```python
from build123d import *

# Parameters (mm, degrees)
SKETCH1_R           = 60
BOSS_EXTRUDE1_DEPTH = 9.652
SKETCH2_R           = 4
BOSS_EXTRUDE2_DEPTH = 25.4
SKETCH3_R           = 60
BOSS_EXTRUDE3_DEPTH = 20
SKETCH5_R           = 36
CUT_EXTRUDE1_DEPTH  = 92.807639682
SKETCH6_R           = 47.5
CUT_EXTRUDE2_DEPTH  = 10
FILLET1_R           = 2.54


with BuildPart() as part:
    # Sketch1 → Boss-Extrude1 (new body)
    with BuildSketch(Plane(origin=(0, 0, 0), x_dir=(1, 0, 0), z_dir=(0, 1, 0))):
        with Locations(Location((0, 0, 0), (0, 0, 270))):
            Circle(SKETCH1_R)
        with BuildLine():
            ThreePointArc((-10.16, 30.080506977), (0, 22.86), (10.16, 30.080506977))
            ThreePointArc((10.16, 30.080506977), (15.875, 27.49630657), (20.970483201, 23.839071591))
            ThreePointArc((20.970483201, 23.839071591), (19.797340731, 11.43), (31.130483201, 6.241435386))
            ThreePointArc((31.130483201, 6.241435386), (31.75, 0), (31.130483201, -6.241435386))
            ThreePointArc((31.130483201, -6.241435386), (19.797340731, -11.43), (20.970483201, -23.839071591))
            ThreePointArc((20.970483201, -23.839071591), (15.875, -27.49630657), (10.16, -30.080506977))
            ThreePointArc((10.16, -30.080506977), (0, -22.86), (-10.16, -30.080506977))
            ThreePointArc((-10.16, -30.080506977), (-15.875, -27.49630657), (-20.970483201, -23.839071591))
            ThreePointArc((-20.970483201, -23.839071591), (-19.797340731, -11.43), (-31.130483201, -6.241435386))
            ThreePointArc((-31.130483201, -6.241435386), (-31.75, 0), (-31.130483201, 6.241435386))
            ThreePointArc((-31.130483201, 6.241435386), (-19.797340731, 11.43), (-20.970483201, 23.839071591))
            ThreePointArc((-20.970483201, 23.839071591), (-15.875, 27.49630657), (-10.16, 30.080506977))
        make_face(mode=Mode.SUBTRACT)
    extrude(amount=BOSS_EXTRUDE1_DEPTH)

    # Sketch2 → Boss-Extrude2 (add)
    with BuildSketch(Plane(origin=(0, 9.652, 0), x_dir=(1, 0, 0), z_dir=(0, 1, 0))):
        with Locations(Location((0, 45, 0), (0, 0, 270))):
            Circle(SKETCH2_R)
        with Locations(Location((38.97114317, -22.5, 0), (0, 0, 270))):
            Circle(SKETCH2_R)
        with Locations(Location((-38.97114317, -22.5, 0), (0, 0, 270))):
            Circle(SKETCH2_R)
    extrude(amount=BOSS_EXTRUDE2_DEPTH)

    # Sketch3 → Boss-Extrude3 (add)
    with BuildSketch(Plane(origin=(0, 35.052, 0), x_dir=(1, 0, 0), z_dir=(0, 1, 0))):
        with Locations(Location((0, 0, 0), (0, 0, 270))):
            Circle(SKETCH3_R)
    extrude(amount=BOSS_EXTRUDE3_DEPTH)

    # Sketch5 → Cut-Extrude1 (cut, through all)
    with BuildSketch(Plane.XZ.offset(-35.052)):
        with Locations(Location((0, 0, 0), (0, 0, 270))):
            Circle(SKETCH5_R)
    extrude(amount=-CUT_EXTRUDE1_DEPTH, mode=Mode.SUBTRACT)

    # Sketch6 → Cut-Extrude2 (cut)
    with BuildSketch(Plane(origin=(0, 55.052, 0), x_dir=(1, 0, 0), z_dir=(0, 1, 0))):
        with Locations(Location((0, 0, 0), (0, 0, 270))):
            Circle(SKETCH6_R)
    extrude(amount=-CUT_EXTRUDE2_DEPTH, mode=Mode.SUBTRACT)

    # Fillet1
    fillet1_edges = [part.edges().sort_by_distance(p)[0] for p in [
        (-10.16, 4.826, 30.080506977),
        (10.16, 4.826, 30.080506977),
        (20.970483201, 4.826, 23.839071591),
        (31.130483201, 4.826, 6.241435386),
        (31.130483201, 4.826, -6.241435386),
        (20.970483201, 4.826, -23.839071591),
        (10.16, 4.826, -30.080506977),
        (-10.16, 4.826, -30.080506977),
        (-20.970483201, 4.826, -23.839071591),
        (-31.130483201, 4.826, -6.241435386),
        (-31.130483201, 4.826, 6.241435386),
        (-20.970483201, 4.826, 23.839071591),
    ]]
    fillet(fillet1_edges, radius=FILLET1_R)


solid = part.part
```
For this review, take the finished solid that the model builds, in its own axes (mm). A direction names the side the tool comes from. Coordinates: 2 decimals unless noted, no trailing zeros. Order: outer loops, then holes, each group sorted by start corner. A loop starts at its lowest first (then second) coordinate and runs counter-clockwise, first axis right, second up. Notation, with made-up numbers: (75.25, 24) -> (89.25, 24) arc R9 cw to (89.25, 28) -> close; hole circle Ø11 at (-1.5, -26.75). An arc over 180 degrees is marked (long way). Answer as CSV lines item,"result".
Q1. We need section D-D (x = -26.5). State the section outline as (y, z) points, plus the area to 3 significant figures.
Model answer:
outline,"(0, -53.83) -> (9.65, -53.83) -> (9.65, -6.37) -> (0, -6.37) -> close; (0, 6.37) -> (9.65, 6.37) -> (9.65, 53.83) -> (0, 53.83) -> close; (35.05, -53.83) -> (55.05, -53.83) -> (55.05, -39.42) -> (45.05, -39.42) -> (45.05, -24.37) -> (35.05, -24.37) -> close; (35.05, 24.37) -> (45.05, 24.37) -> (45.05, 39.42) -> (55.05, 39.42) -> (55.05, 53.83) -> (35.05, 53.83) -> close"
area,"1,790 mm2"
Q2. For faces 1 (the face through (-2.4, 22.2, -48.2)), 2 (the face through (-0.16, 4.76, -22.86)), 3 (the face through (10.81, 39.98, -34.34)), list the 3-axis set-ups (+Z, -Z, +X, -X, +Y, -Y) from which the entire face can be reached by the end or side of a thin tool; tool diameter is ignored.
Model answer:
face 1,"none"
face 2,"+Y, -Y"
face 3,"+Y"
Q3. Clearance check with flat-ended pins moving along their axes: pin 1 Ø1.5 at (y, z) = (49.5, 45.5) entering from +X; pin 2 Ø10 at (y, z) = (24, 14.5) entering from -X; pin 3 Ø4 at (x, y) = (-20.5, 45) entering from +Z. State where each tip first meets the part, or that it passes through.
Model answer:
pin 1,"stops at x = 39.97"
pin 2,"stops at x = -41.62"
pin 3,"stops at z = 57.08"
Q4. We need section C-C (z = 0). State the section outline as (x, y) points.
Model answer:
outline,"(-60, 0) -> (-31.75, 0) -> (-31.75, 9.65) -> (-60, 9.65) -> close; (-60, 35.05) -> (-36, 35.05) -> (-36, 45.05) -> (-47.5, 45.05) -> (-47.5, 55.05) -> (-60, 55.05) -> close; (31.75, 0) -> (60, 0) -> (60, 9.65) -> (31.75, 9.65) -> close; (36, 35.05) -> (60, 35.05) -> (60, 55.05) -> (47.5, 55.05) -> (47.5, 45.05) -> (36, 45.05) -> close"
Q5. Draft analysis for pull direction X (two halves, no side actions). For faces 4 (the face through (18.1, 55.052, 44.2)), 5 (the face through (-38.795, 22.174, 18.504)), 6 (the face through (2.64, 4.76, -59.94)), state which applies: released by +X, released by -X, zero draft, split by the parting line, or undercut.
Model answer:
face 4,"zero draft"
face 5,"undercut"
face 6,"split by the parting line"
Q6. Wall thickness on line 1 along X through (y, z) = (5, 0); line 2 along Y through (x, z) = (-25.5, -53.5); line 3 along X through (y, z) = (38, 0): over which ranges is each line inside the solid? List them lowest first. Write a range as [from, to].
Model answer:
line 1,"x = [-60, -31.75], [31.75, 60]"
line 2,"y = [0, 9.65], [35.05, 55.05]"
line 3,"x = [-60, -36], [36, 60]"
Q7. We need section A-A (x = 0). State the section outline as (y, z) points.
Model answer:
outline,"(0, -60) -> (9.65, -60) -> (9.65, -49) -> (35.05, -49) -> (35.05, -60) -> (55.05, -60) -> (55.05, -47.5) -> (45.05, -47.5) -> (45.05, -36) -> (35.05, -36) -> (35.05, -41) -> (9.65, -41) -> (9.65, -22.86) -> (0, -22.86) -> close; (0, 22.86) -> (9.65, 22.86) -> (9.65, 60) -> (0, 60) -> close; (35.05, 36) -> (45.05, 36) -> (45.05, 47.5) -> (55.05, 47.5) -> (55.05, 60) -> (35.05, 60) -> close"
Q8. We need section B-B (z = 31). State the section outline as (x, y) points.
Model answer:
outline,"(-51.37, 0) -> (51.37, 0) -> (51.37, 9.65) -> (-51.37, 9.65) -> close; (-51.37, 35.05) -> (-18.3, 35.05) -> (-18.3, 45.05) -> (-35.99, 45.05) -> (-35.99, 55.05) -> (-51.37, 55.05) -> close; (18.3, 35.05) -> (51.37, 35.05) -> (51.37, 55.05) -> (35.99, 55.05) -> (35.99, 45.05) -> (18.3, 45.05) -> close"
